```python
from build123d import *

# Parameters (mm, degrees)
F0_R          = 2.5
F0_R_2        = 1.5
F4_DEPTH      = 15
F4_DEPTH_BACK = 10
F6_R          = 2.55
F6_R_2        = 2.5
F7_DEPTH      = 0.25
F10_R         = 5
F10_R_2       = 1.5
F11_DEPTH     = 1.2
F14_R         = 1.5
F15_DEPTH     = 2
F3_R          = 1
F18_R         = 1
F20_DEPTH     = 14


with BuildPart() as f4:
    # F0 (on Top) → F4 (new body, two sides)
    with BuildSketch(Plane.XY) as f4_sk:
        Circle(F0_R)
        Circle(F0_R_2, mode=Mode.SUBTRACT)
    extrude(amount=F4_DEPTH)
    extrude(f4_sk.sketch, amount=-F4_DEPTH_BACK)

    # F6 (on face) → F7 (join)
    with BuildSketch(Plane.XY.offset(15)):
        Circle(F6_R)
        Circle(F6_R_2, mode=Mode.SUBTRACT)
    extrude(amount=-F7_DEPTH)

    # F10 (on Top) → F11 (join)
    with BuildSketch(Plane.XY):
        Circle(F10_R)
        Circle(F10_R_2, mode=Mode.SUBTRACT)
    extrude(amount=F11_DEPTH)

    # F12 (on Front) → F13 (revolve)
    with BuildSketch(Plane.XZ):
        with BuildLine():
            Line((5, 0), (2.5, 0))
            Line((2.5, 0), (2.5, -10))
            Line((2.5, -10), (8.7983487174, -10))
            add(Edge.make_bspline(
                [(5, 0), (5.0383992493, -4.4832699932), (6.3285781071, -8.5749803111), (8.7983487174, -10)],
                knots=[0, 0, 0, 0, 10.6970768427, 10.6970768427, 10.6970768427, 10.6970768427], degree=3))
        make_face()
    revolve(axis=Axis((0, 0, -7.6235234737), (0, 0, -1)))

    # F14 (on face) → F15 (join)
    with BuildSketch(Plane(origin=(0, 0, -10), x_dir=(1, 0, 0), z_dir=(0, 0, -1))):
        Circle(F14_R)
    extrude(amount=-F15_DEPTH)

    # F16: sweep along a path in F1
    with BuildLine(Plane.XZ) as f16_path:
        Line((0, -6.4742463656), (7.6604444312, -0.0463702687))
    # F3 (on line) → F16 (sweep, cut)
    with BuildSketch(Plane(origin=(4.4725004233, 0, 3.7528734556), x_dir=(0, 1, 0), z_dir=(0.7660444431, 0, 0.6427876097))):
        with Locations((0, -4.96)):
            Circle(F3_R)
    sweep(path=f16_path.line, mode=Mode.SUBTRACT)

    # F19: sweep along a path in F1
    with BuildLine(Plane.XZ) as f19_path:
        Line((0, -6.4742463656), (-7.6604444312, -0.0463702687))
    # F18 (on line) → F19 (sweep, cut)
    with BuildSketch(Plane(origin=(-4.4725004233, 0, 3.7528734556), x_dir=(0, -1, 0), z_dir=(-0.7660444431, 0, 0.6427876097))):
        with Locations((0, -4.9955216867)):
            Circle(F18_R)
    sweep(path=f19_path.line, mode=Mode.SUBTRACT)

    # F20 (add): a face of the model
    f20_faces = [f4.faces().sort_by_distance(p)[0] for p in [
        (-4.8585786438, 0, 1.2),
    ]]
    extrude(f20_faces, amount=F20_DEPTH)


solid = f4.part
```
Read the model definition and answer for the solid it produces. Units are mm, in the model's axes. A direction names the side the tool comes from. Round coordinates to 2 decimals unless told otherwise and drop trailing zeros. Write each loop counter-clockwise with the first axis right and the second up, starting at its lowest first coordinate (ties: lowest second). Pieces come first, ordered by that corner, then holes. Notation, with made-up numbers: (-13, 45.5) -> (31, 45.5) arc R22 ccw to (31, 69.5) -> close; hole circle Ø10 at (65, -24). An arc over 180 degrees is marked (long way). Answer in a Markdown table with one row per item. Add a question column.
1) Consider line 1 (Y direction, x = 0, z = 15.1); line 2 (X direction, y = -4.25, z = -8.25); line 3 (X direction, y = -0.25, z = 3.5). Determine where each line is inside the solid, lowest interval first.
2) Find section B-B, the plane y = 0.5. State how many separate pieces and enclosed holes the cut face has, and give its area (3 significant figures).
3) Determine the mould class of faces 1 (the face through (0, 0, -8)), 2 (the face through (-1.08, -4.88, 7.49)), 3 (the face through (2, -2, 15.2)) for opening direction Y: pulls with the +Y half, pulls with the -Y half, needs draft (parallel to the pull), parting line crosses it, or undercut.
4) Given P1, Ø4, axis at y = 2.5, z = 8.5, coming from the +X side; P2, Ø8, axis at x = -5.5, z = 5.5, coming from the +Y side; P3, Ø3, axis at x = -6, z = -2.5, coming from the -Y side, each flat-ended and moving along its own axis, determine where each tip first touches the part or whether it passes through.
5) Which of the six approach directions +Z, -Z, +X, -X, +Y, -Y give full straight-line access (tool end or side, diameter ignored) to faces 4 (the face through (-3.926, 0.217, -4.501)), 5 (the face through (-1.5, 0.07, 3.34))?
6) Find section A-A, the plane z = 4.5. Determine the outline of the cut face in (x, y), and give its area (3 significant figures).
Findings below:
| question | item | result |
|---|---|---|
| 1 | line 1 | -5 to -2.5, 2.5 to 5 |
| 1 | line 2 | -5.59 to 5.59 |
| 1 | line 3 | -4.99 to -1.48, 1.48 to 4.99 |
| 2 | separate pieces | 3 |
| 2 | enclosed holes | 0 |
| 2 | area | 188 mm² |
| 3 | face 1 | undercut |
| 3 | face 2 | parting line crosses it |
| 3 | face 3 | needs draft |
| 4 | P1 | x = 4.97 |
| 4 | P2 | y = 4.77 |
| 4 | P3 | y = -2.55 |
| 5 | face 4 | none |
| 5 | face 5 | +Z |
| 6 | outline | circle Ø10 at (0, 0); hole circle Ø3 at (0, 0) |
| 6 | area | 71.5 mm² |
